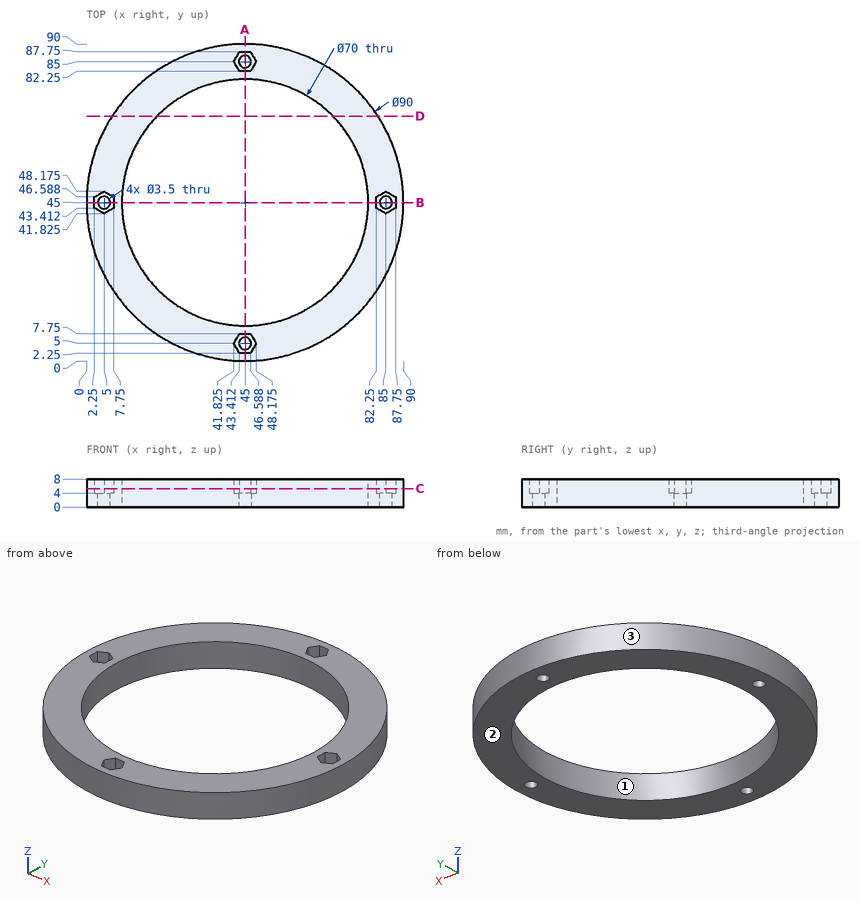
Print and shaded views of the part. All mm, measured from the part's lowest x, y and z. Coordinates: 2 decimals unless noted, no trailing zeros. Write each loop counter-clockwise with the first axis right and the second up, starting at its lowest first coordinate (ties: lowest second). Pieces come first, ordered by that corner, then holes.
(1) Cut at C-C, the plane z = 5.25. Count the separate pieces of the cut face and the enclosed holes in it, and give its area (3 significant figures).
(2) Cut at A-A, the plane x = 45. List the corners of the cut face in (y, z).
(3) Cut at D-D, the plane y = 69.5. List the corners of the cut face in (x, z) (1 decimal), and give its area (3 significant figures).
(4) Two-plate mould, pull along X, no slides. Class the marked faces 1, 2 and 3: +X half, -X half, draft (parallel to the pull), parting line (faces both ways), or undercut.
(5) Drill centre lines: probe 1 along Y at (x, z) = (45, 1.95); probe 2 along Y at (x, z) = (45, 6); probe 3 along X at (y, z) = (48, 7.25) (1 decimal). Where is each one in solid material? Low to high.
(6) Flat gauge pins, fed straight in: pin 1 (2.5 mm diameter, centred on x = 44.5, z = 5, fed in from +Y); pin 2 (1 mm diameter, centred on x = 52.5, z = 6.5, fed in from +Y); pin 3 (1.6 mm diameter, centred on y = 46, z = 5.5, fed in from +X). Where does each tip first touch, or does it go through?
Geometry says:
1. separate pieces: 1
1. enclosed holes: 5
1. area: 2,410 mm2
2. outline: (0, 0) - (3.25, 0) - (3.25, 4) - (2.25, 4) - (2.25, 8) - (0, 8) - close; (6.75, 0) - (10, 0) - (10, 8) - (7.75, 8) - (7.75, 4) - (6.75, 4) - close; (80, 0) - (83.25, 0) - (83.25, 4) - (82.25, 4) - (82.25, 8) - (80, 8) - close; (86.75, 0) - (90, 0) - (90, 8) - (87.75, 8) - (87.75, 4) - (86.75, 4) - close
3. outline: (7.3, 0) - (20, 0) - (20, 8) - (7.3, 8) - close; (70, 0) - (82.7, 0) - (82.7, 8) - (70, 8) - close
3. area: 204 mm2
4. face 1: undercut
4. face 2: draft
4. face 3: parting line
5. probe 1: y = 0 to 3.25, 6.75 to 10, 80 to 83.25, 86.75 to 90
5. probe 2: y = 0 to 2.25, 7.75 to 10, 80 to 82.25, 87.75 to 90
5. probe 3: x = 0.1 to 4.7, 5.3 to 10.1, 79.9 to 84.7, 85.3 to 89.9
6. pin 1: stops at y = 90
6. pin 2: stops at y = 89.45
6. pin 3: stops at x = 90
